Study the drawing (mm; zero at the part's minimum x, y, z) and answer. A direction names the side the tool comes from. Coordinates: 2 decimals unless noted, no trailing zeros. Order: outer loops, then holes, each group sorted by start corner. A loop starts at its lowest first (then second) coordinate and runs counter-clockwise, first axis right, second up.
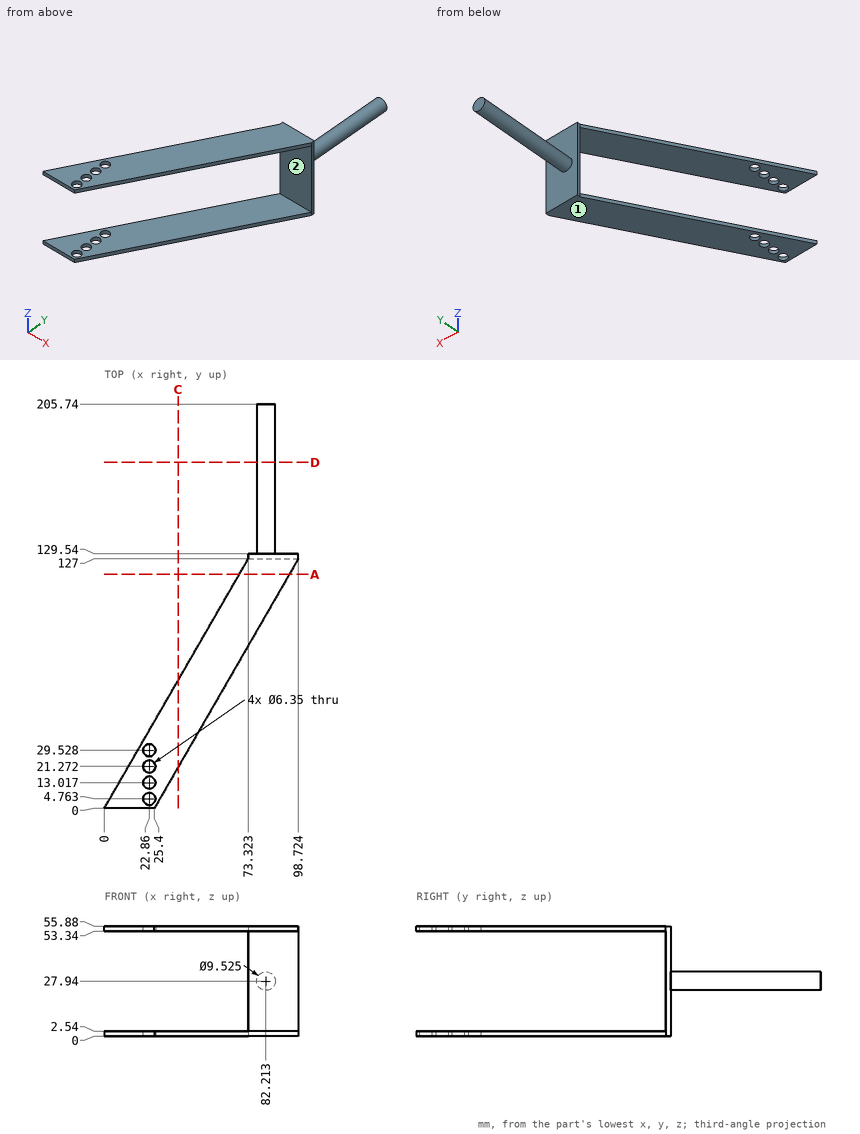
(1) Find section C-C on x = 37.5. Determine the outline of the cut face in (y, z).
(2) Find section D-D on y = 176. Determine the outline of the cut face in (x, z) (1 decimal).
(3) A tool of negligible diameter and unlimited length cuts with its end or side. For the marked faces 1 and 2, from which of +Z, -Z, +X, -X, +Y, -Y can it reach the whole face along a straight path? Write none if from no direction.
(4) Find the intervals of material crossed by probe 1 along Z at (x, y) = (67.5, 90); probe 2 along Y at (x, z) = (22, 55) (1 decimal); probe 3 along X at (y, z) = (128, 9), in increasing order.
(5) Find section A-A on y = 119. Determine the outline of the cut face in (x, z) (1 decimal), then the cut area to 3 significant figures.
(6) Given pin 1 Ø20.5 at (x, z) = (92, 24) entering from -Y; pin 2 Ø5.5 at (x, y) = (22.86, 13.02) entering from +Z; pin 3 Ø0.8 at (y, z) = (128.5, 19.5) entering from -X, each flat-ended and moving along its own axis, determine where each tip first touches the part or whether it passes through.
Resolved:
1. outline: (20.96, 0) - (64.95, 0) - (64.95, 2.54) - (20.96, 2.54) - close; (20.96, 53.34) - (64.95, 53.34) - (64.95, 55.88) - (20.96, 55.88) - close
2. outline: circle Ø9.5 at (82.2, 27.9)
3. face 1: -Z, +X, -X, +Y, -Y
3. face 2: +X, -X, -Y
4. probe 1: z = 0 to 2.54, 53.34 to 55.88
4. probe 2: y = 0 to 1.7, 7.8 to 10, 16.1 to 18.2, 24.3 to 26.5, 32.6 to 38.1
4. probe 3: x = 73.32 to 98.72
5. outline: (68.7, 0) - (94.1, 0) - (94.1, 2.5) - (68.7, 2.5) - close; (68.7, 53.3) - (94.1, 53.3) - (94.1, 55.9) - (68.7, 55.9) - close
5. area: 129 mm2
6. pin 1: stops at y = 127
6. pin 2: passes through
6. pin 3: stops at x = 73.32
